```python
from build123d import *

# Parameters (mm, degrees)
F0_R     = 38.1
F1_DEPTH = 34.798
F2_T     = -2.54


# Not quite as in the source:
# - a fillet or chamfer that OpenCascade refuses, or shapes differently, is made with other operations: its cross-section is extruded or revolved along the edge and cut away or added
# - the program builds the solid bodies; features that only make, move or delete a surface that nothing else refers to are left out


with BuildPart() as f1:
    # F0 (on Top) → F1 (new body, symmetric)
    with BuildSketch(Plane.XY):
        Circle(F0_R)
    extrude(amount=F1_DEPTH, both=True)

    # F2
    f2_openings = [f1.faces().sort_by_distance(p)[0] for p in [
        (0, 0, 34.798),
    ]]
    offset(amount=F2_T, openings=f2_openings)

    # F3: fillet of radius 10.4245741623 on 1 edges, made by hand

    # F3_s1 → F3_t2 (revolve, cut)
    with BuildSketch(Plane.XZ):
        with BuildLine():
            ThreePointArc((38.1, 27.9785251856), (37.4443836777, 31.617097596), (35.56, 34.798))
            Line((35.56, 34.798), (38.1, 34.798))
            Line((38.1, 34.798), (38.1, 27.9785251856))
        make_face()
    revolve(axis=Axis((0, 0, 34.798), (0, 0, 1)), mode=Mode.SUBTRACT)


solid = f1.part
```
Verification items for the finished model (mm, model axes). Give positions to 0.01 mm unless a question says otherwise; leave off trailing zeros. Loops run counter-clockwise (first coordinate to the right, second up) from the corner with the lowest first, then second, coordinate; pieces in that order, holes last. Notation, with made-up numbers: M 69.5,26 L 77.5,26 A23 ccw 77.5,60 Z; hole C 49,40.5 d10. An arc over 180 degrees is marked long. Return JSON: item names as keys, results as strings.
1) Gauge pin test, flat ends, axial feed: P1, Ø12, axis at x = -3.5, z = -19, coming from the +Y side; P2, Ø1.5, axis at y = -12.5, z = 7.5, coming from the +X side; P3, Ø8, axis at x = 17.5, y = 17, coming from the +Z side. Record the tip position at first contact, or that the pin passes through.
Findings:
{"P1": "stops at y = 38.1", "P2": "stops at x = 36.24", "P3": "stops at z = -32.26"}
2) Mould release check, pull along Y, two halves, no side actions. Record for faces 1 (the cylindrical face through (-7.709, -34.714, 1.739)), 2 (the flat face through (-1, 1, -34.798)), 3 (the cylindrical face through (-30.235, -23.183, -2.97)): released by +Y, released by -Y, zero draft, split by the parting line, or undercut.
Findings:
{"face 1": "undercut", "face 2": "zero draft", "face 3": "split by the parting line"}
3) Material ranges on L1, parallel to Y at x = 0, z = -1; L2, parallel to Z at x = 11, y = 13; L3, parallel to Y at x = 30.5, z = 15, recorded low to high. Write a range as [from, to].
Findings:
{"L1": "y = [-38.1, -35.56], [35.56, 38.1]", "L2": "z = [-34.8, -32.26]", "L3": "y = [-22.83, -18.28], [18.28, 22.83]"}
4) Section check A-A, the plane x = 0. Enter the section's corners in (y, z), and give its area (3 significant figures).
Findings:
{"outline": "M -38.1,-34.8 L 38.1,-34.8 L 38.1,27.98 A10.42 ccw 35.56,34.8 L 35.56,-32.26 L -35.56,-32.26 L -35.56,34.8 A10.42 ccw -38.1,27.98 Z", "area": "523 mm2"}
5) Section check C-C, the plane z = -25. Enter the section's corners in (x, y).
Findings:
{"outline": "C 0,0 d76.2; hole C 0,0 d71.12"}
